Geometry check sheet. Reference: the model listing, model coordinates, mm. Round coordinates to 2 decimals unless told otherwise and drop trailing zeros. Order: outer loops, then holes, each group sorted by start corner. A loop starts at its lowest first (then second) coordinate and runs counter-clockwise, first axis right, second up. Notation, with made-up numbers: (46, 27.25) - (54, 27.25) arc R10 cw to (54, 31.25) - close; hole circle Ø10 at (31.25, 40). An arc over 180 degrees is marked (long way). Write each question's results on one line, items separated by ' | '.
```python
from build123d import *

# Parameters (mm, degrees)
CROQUIS1_W              = 150
CROQUIS1_H              = 200
CROQUIS1_W_2            = 5
CROQUIS1_H_2            = 30
SALIENTE_EXTRUIR1_DEPTH = 5
REDONDEO1_R             = 30
CORTAR_EXTRUIR1_REACH   = 281.518
CROQUIS2_R              = 2


with BuildPart() as part:
    # Croquis1 → Saliente-Extruir1 (new body)
    with BuildSketch(Plane.XY):
        with Locations((-167.295474365, 39.278017241)):
            Rectangle(CROQUIS1_W, CROQUIS1_H)
        with Locations((-167.295474365, 104.278017241)):
            Rectangle(CROQUIS1_W_2, CROQUIS1_H_2, mode=Mode.SUBTRACT)
    extrude(amount=SALIENTE_EXTRUIR1_DEPTH)

    # Redondeo1
    redondeo1_edges = [part.edges().sort_by_distance(p)[0] for p in [
        (-242.295474365, 139.278017241, 2.5),
        (-92.295474365, 139.278017241, 2.5),
        (-92.295474365, -60.721982759, 2.5),
        (-242.295474365, -60.721982759, 2.5),
    ]]
    fillet(redondeo1_edges, radius=REDONDEO1_R)

    # Croquis2 → Cortar-Extruir1 (cut, up to next)
    with BuildSketch(Plane.XY.offset(5), mode=Mode.PRIVATE) as cortar_extruir1_sk1:
        with Locations((-144.795474365, 111.778017241)):
            Circle(CROQUIS2_R)
    cortar_extruir1_tool1 = extrude(cortar_extruir1_sk1.sketch, amount=-CORTAR_EXTRUIR1_REACH, mode=Mode.PRIVATE) & part.part
    # Croquis2 → Cortar-Extruir1 (cut, up to next)
    with BuildSketch(Plane.XY.offset(5), mode=Mode.PRIVATE) as cortar_extruir1_sk2:
        with Locations((-189.795474365, 111.778017241)):
            Circle(CROQUIS2_R)
    cortar_extruir1_tool2 = extrude(cortar_extruir1_sk2.sketch, amount=-CORTAR_EXTRUIR1_REACH, mode=Mode.PRIVATE) & part.part
    # Croquis2 → Cortar-Extruir1 (cut, up to next)
    with BuildSketch(Plane.XY.offset(5), mode=Mode.PRIVATE) as cortar_extruir1_sk3:
        with Locations((-189.795474365, 96.778017241)):
            Circle(CROQUIS2_R)
    cortar_extruir1_tool3 = extrude(cortar_extruir1_sk3.sketch, amount=-CORTAR_EXTRUIR1_REACH, mode=Mode.PRIVATE) & part.part
    # Croquis2 → Cortar-Extruir1 (cut, up to next)
    with BuildSketch(Plane.XY.offset(5), mode=Mode.PRIVATE) as cortar_extruir1_sk4:
        with Locations((-144.795474365, 96.778017241)):
            Circle(CROQUIS2_R)
    cortar_extruir1_tool4 = extrude(cortar_extruir1_sk4.sketch, amount=-CORTAR_EXTRUIR1_REACH, mode=Mode.PRIVATE) & part.part
    add(cortar_extruir1_tool1.solids().sort_by_distance((-144.795474, 111.778017, 5))[0], mode=Mode.SUBTRACT)
    add(cortar_extruir1_tool2.solids().sort_by_distance((-189.795474, 111.778017, 5))[0], mode=Mode.SUBTRACT)
    add(cortar_extruir1_tool3.solids().sort_by_distance((-189.795474, 96.778017, 5))[0], mode=Mode.SUBTRACT)
    add(cortar_extruir1_tool4.solids().sort_by_distance((-144.795474, 96.778017, 5))[0], mode=Mode.SUBTRACT)


solid = part.part
```
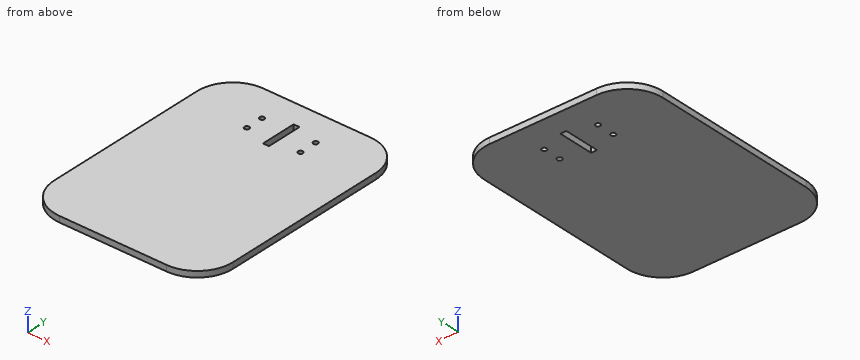
(1) Section check A-A (z = 3.25). Record the cut outline in (x, y), then the cut area to 3 significant figures.
Answers follow:
outline: (-242.3, -30.72) arc R30 ccw to (-212.3, -60.72) - (-122.3, -60.72) arc R30 ccw to (-92.3, -30.72) - (-92.3, 109.28) arc R30 ccw to (-122.3, 139.28) - (-212.3, 139.28) arc R30 ccw to (-242.3, 109.28) - close; hole circle Ø4 at (-189.8, 96.78); hole circle Ø4 at (-189.8, 111.78); hole (-169.8, 89.28) - (-164.8, 89.28) - (-164.8, 119.28) - (-169.8, 119.28) - close; hole circle Ø4 at (-144.8, 96.78); hole circle Ø4 at (-144.8, 111.78) | area: 29,000 mm²
(2) Section check C-C (x = -223). Record the cut outline in (y, z).
Answers follow:
outline: (-58.75, 0) - (137.3, 0) - (137.3, 5) - (-58.75, 5) - close
(3) Material ranges on line 1 (Y direction, x = -167, z = 4.1); line 2 (Y direction, x = -144, z = 1.45); line 3 (Y direction, x = -121.5, z = 3.45), recorded low to high.
Answers follow:
line 1: -60.72 to 89.28, 119.28 to 139.28 | line 2: -60.72 to 94.94, 98.61 to 109.94, 113.61 to 139.28 | line 3: -60.71 to 139.27
(4) Section check B-B (y = -48). Record the cut outline in (x, z).
Answers follow:
outline: (-236.82, 0) - (-97.77, 0) - (-97.77, 5) - (-236.82, 5) - close
